Could you check a few things on this model? Use its own coordinates, in mm. A direction names the side the tool comes from. Coordinates: 2 decimals unless noted, no trailing zeros. Order: outer loops, then holes, each group sorted by start corner. A loop starts at its lowest first (then second) coordinate and runs counter-clockwise, first axis right, second up. Notation, with made-up numbers: (-27.75, 45) -> (-22.75, 45) arc R17 ccw to (-22.75, 61) -> close; hole circle Ø7 at (-16.5, 83.25). An arc over 180 degrees is marked (long way). Return JSON: item names as keys, results as strings. Group by question number.
from build123d import *

# Parameters (mm, degrees)
F0_W     = 1016
F0_H     = 774.7
F1_DEPTH = 19.05
F3_DEPTH = 1016.001
F4_W     = 952.1952
F4_H     = 545.7952
F5_DEPTH = 19.051
F7_DEPTH = 1.5875
F9_DEPTH = 1016.001


with BuildPart() as f1:
    # F0 (on Front) → F1 (new body)
    with BuildSketch(Plane.XZ):
        with Locations((-46.856156, 110.373389)):
            Rectangle(F0_W, F0_H)
    extrude(amount=-F1_DEPTH)

    # F2 (on face) → F3 (cut, through all)
    with BuildSketch(Plane.YZ.offset(461.143844)):
        Polygon((19.05, -269.085843), (0, -276.976611), (19.05, -276.976611), align=None)
    extrude(amount=-F3_DEPTH, mode=Mode.SUBTRACT)

    # F4 (on face) → F5 (cut, through all)
    with BuildSketch(Plane.XZ):
        with Locations((-46.856156, 160.995589)):
            Rectangle(F4_W, F4_H)
    extrude(amount=-F5_DEPTH, mode=Mode.SUBTRACT)

    # F6 (on face) → F7 (cut)
    with BuildSketch(Plane.XZ):
        Polygon((276.993844, 472.323389), (-46.856156, 472.323389), (-370.706156, 472.323389), (-370.706156, 433.893189), (276.993844, 433.893189), align=None)
        Polygon((276.993844, -111.902011), (-370.706156, -111.902011), (-370.706156, -150.332211), (-46.856156, -150.332211), (276.993844, -150.332211), align=None)
    extrude(amount=-F7_DEPTH, mode=Mode.SUBTRACT)

    # F8 (on face) → F9 (cut, through all)
    with BuildSketch(Plane.YZ.offset(461.143844)):
        Polygon((19.05, 497.723389), (0, 497.723389), (0, 489.832621), align=None)
    extrude(amount=-F9_DEPTH, mode=Mode.SUBTRACT)


solid = f1.part
Q1. I want a section at A-A on x = -82.5. Please give me the cut outline in (y, z), and give its area (3 significant figures).
Q2. On a 3-axis mill with a long thin cutter (end or side, diameter ignored), from which of +Z, -Z, +X, -X, +Y, -Y can I reach the whole of each face in a straight line? I mean faces 3 (the flat face through (-51, 1.588, -131)), 4 (the flat face through (-49, 0, -176)). Say none if no direction works.
Q3. I'm going to push flat-ended pins straight in: pin 1 Ø4 at (x, y) = (-379.5, 16.5) entering from -Z; pin 2 Ø0.8 at (x, y) = (-200, 1) entering from +Z; pin 3 Ø5.5 at (x, y) = (-144, 7.5) entering from -Z. Where does each tip first touch, or does it pass through?
Q4. I want a section at D-D on x = -419.5. Please give me the cut outline in (y, z).
Q5. I want a section at B-B on z = 400.5. Please give me the cut outline in (x, y), and give its area (3 significant figures).
Q6. I want a section at C-C on y = 13.5. Please give me the cut outline in (x, z), and give its area (3 significant figures).
Q7. I need wall thicknesses on line 1 along X through (y, z) = (14, 56.5); line 2 along Z through (x, y) = (-379, 3.5); line 3 along Z through (x, y) = (-282, 1). Which ranges of each line are inside material? Lowest first, please. Write a range as from..to.
Q8. We'd pull the mould along Z, two halves only. Please class faces 1 (the flat face through (-49, 19.05, -139)), 2 (the flat face through (-51, 1.588, 453)): pulls with the +Z half, pulls with the -Z half, needs draft (parallel to the pull), parting line crosses it, or undercut.
Response values:
{
 "1": {"outline": "(0, -276.98) -> (19.05, -269.09) -> (19.05, -111.9) -> (1.59, -111.9) -> (1.59, -150.33) -> (0, -150.33) -> close; (0, 472.32) -> (1.59, 472.32) -> (1.59, 433.89) -> (19.05, 433.89) -> (19.05, 497.72) -> (0, 489.83) -> close", "area": "4,090 mm²"},
 "2": {"face 3": "-Y", "face 4": "+Z, -Z, +X, -X, -Y"},
 "3": {"pin 1": "stops at z = -270.97", "pin 2": "stops at z = 490.41", "pin 3": "stops at z = -275.01"},
 "4": {"outline": "(0, -276.98) -> (19.05, -269.09) -> (19.05, -111.9) -> (0, -111.9) -> close; (0, 433.89) -> (19.05, 433.89) -> (19.05, 497.72) -> (0, 489.83) -> close"},
 "5": {"outline": "(-554.86, 0) -> (-522.95, 0) -> (-522.95, 19.05) -> (-554.86, 19.05) -> close; (429.24, 0) -> (461.14, 0) -> (461.14, 19.05) -> (429.24, 19.05) -> close", "area": "1,220 mm²"},
 "6": {"outline": "(-554.86, -271.38) -> (461.14, -271.38) -> (461.14, 495.42) -> (-554.86, 495.42) -> close; hole (-522.95, -111.9) -> (429.24, -111.9) -> (429.24, 433.89) -> (-522.95, 433.89) -> close", "area": "259,000 mm²"},
 "7": {"line 1": "x = -554.86..-522.95, 429.24..461.14", "line 2": "z = -275.53..-111.9, 433.89..491.28", "line 3": "z = -276.56..-150.33, 472.32..490.25"},
 "8": {"face 1": "needs draft", "face 2": "undercut"}
}
